from build123d import *

# Parameters (mm, degrees)
CYLINDER074_R             = 11
CYLINDER074_DEPTH         = 10
CYLINDER075_R             = 8
CYLINDER075_DEPTH         = 28
CYLINDER076_R             = 11
CYLINDER076_DEPTH         = 10
CYLINDER083_R             = 1.7
CYLINDER083_DEPTH         = 21
BOX019_W                  = 23
BOX019_H                  = 5.2
BOX019_DEPTH              = 3
PRISM012_DEPTH            = 3
FUSION068_ROLL_ANGLE      = 180
FUSION068_PLACEMENT_ANGLE = 90
EXTRUDE034_DEPTH          = 275
CYLINDER085_R             = 4
CYLINDER085_DEPTH         = 70
PRISM013_DEPTH            = 6
FUSION069_PITCH_ANGLE     = -90
FUSION069_PLACEMENT_ANGLE = -90
CYLINDER073_R             = 11
CYLINDER073_DEPTH         = 10
BOX018_W                  = 34
BOX018_H                  = 24
BOX018_DEPTH              = 6
CYLINDER081_R             = 2.9
CYLINDER081_DEPTH         = 2
CYLINDER082_R             = 2.9
CYLINDER082_DEPTH         = 2
CYLINDER084_R             = 7
CYLINDER084_DEPTH         = 3
EXTRUDE032_DEPTH          = 6
FILLET005_R               = 1.6


with BuildPart() as cilindro074:
    # Cylinder074 → Cylinder074 (new body)
    with BuildSketch(Plane(origin=(83, 3, 55), x_dir=(1, 0, 0), z_dir=(0, 1, 0))):
        Circle(CYLINDER074_R)
    extrude(amount=CYLINDER074_DEPTH)


with BuildPart() as cilindro075:
    # Cylinder075 → Cylinder075 (new body)
    with BuildSketch(Plane(origin=(83, -14, 55), x_dir=(1, 0, 0), z_dir=(0, 1, 0))):
        Circle(CYLINDER075_R)
    extrude(amount=CYLINDER075_DEPTH)


with BuildPart() as cilindro076:
    # Cylinder076 → Cylinder076 (new body)
    with BuildSketch(Plane(origin=(83, -3, 55), x_dir=(1, 0, 0), z_dir=(0, -1, 0))):
        Circle(CYLINDER076_R)
    extrude(amount=CYLINDER076_DEPTH)


with BuildPart() as cilindro083:
    # Cylinder083 → Cylinder083 (new body)
    with BuildSketch(Plane.XY.offset(-6)):
        Circle(CYLINDER083_R)
    extrude(amount=CYLINDER083_DEPTH)


with BuildPart() as cubo018:
    # Box019 → Box019 (new body)
    with BuildSketch(Plane(origin=(0, -2.6, 0), x_dir=(1, 0, 0), z_dir=(0, 0, 1))):
        with Locations((11.5, 2.6)):
            Rectangle(BOX019_W, BOX019_H)
    extrude(amount=BOX019_DEPTH)


with BuildPart() as hueco_tornillo004:
    # Prism012 → Prism012 (new body)
    with BuildSketch(Plane.XY):
        Polygon((3, 0), (1.5, 2.598076), (-1.5, 2.598076), (-3, 0), (-1.5, -2.598076), (1.5, -2.598076), align=None)
    extrude(amount=PRISM012_DEPTH)

    # Fusion068: union Cilindro083, Cubo018
    add(cilindro083.part)
    add(cubo018.part)


with BuildPart() as hueco_tornillo004_1:
    # Fusion068 roll: moved
    add(hueco_tornillo004.part.rotate(Axis((0, 0, 0), (1, 0, 0)), FUSION068_ROLL_ANGLE))


with BuildPart() as hueco_tornillo004_2:
    # Fusion068 placement: moved
    add(hueco_tornillo004_1.part.moved(Location((159, 0, 62))).rotate(Axis((159, 0, 62), (0, 0, 1)), FUSION068_PLACEMENT_ANGLE))


with BuildPart() as extrude034:
    # Sketch026 → Extrude034 (new body)
    with BuildSketch(Plane.YZ):
        with BuildLine():
            ThreePointArc((3.10248, -2.60329), (0, 4.05), (-3.10248, -2.60329))
            Line((-3.10248, -2.60329), (-1.888546, -4.05))
            Line((-1.888546, -4.05), (0, -4.05))
            Line((0, -4.05), (1.888546, -4.05))
            Line((3.10248, -2.60329), (1.888546, -4.05))
        make_face()
    extrude(amount=EXTRUDE034_DEPTH)


with BuildPart() as extrude034_1:
    # Extrude034 placement: moved
    add(extrude034.part.moved(Location((0, 0, 71))))


with BuildPart() as cilindro085:
    # Cylinder085 → Cylinder085 (new body)
    with BuildSketch(Plane.XY):
        Circle(CYLINDER085_R)
    extrude(amount=CYLINDER085_DEPTH)


with BuildPart() as tornillo_m010:
    # Prism013 → Prism013 (new body)
    with BuildSketch(Plane.XY):
        Polygon((7.55, 0), (3.775, 6.538492), (-3.775, 6.538492), (-7.55, 0), (-3.775, -6.538492), (3.775, -6.538492), align=None)
    extrude(amount=PRISM013_DEPTH)

    # Fusion069: union Cilindro085
    add(cilindro085.part)


with BuildPart() as tornillo_m010_1:
    # Fusion069 pitch: moved
    add(tornillo_m010.part.rotate(Axis((0, 0, 0), (0, 1, 0)), FUSION069_PITCH_ANGLE))


with BuildPart() as tornillo_m010_2:
    # Fusion069 placement: moved
    add(tornillo_m010_1.part.moved(Location((203, -7, 55))).rotate(Axis((203, -7, 55), (0, 0, 1)), FUSION069_PLACEMENT_ANGLE))


with BuildPart() as fusion065:
    # Cylinder073 → Cylinder073 (new body)
    with BuildSketch(Plane(origin=(83, -3, 55), x_dir=(1, 0, 0), z_dir=(0, -1, 0))):
        Circle(CYLINDER073_R)
    extrude(amount=CYLINDER073_DEPTH)

    # Fusion065: union Cilindro074, Cilindro075, Cilindro076, hueco_tornillo004, Extrude034, Tornillo_M010
    add(cilindro074.part)
    add(cilindro075.part)
    add(cilindro076.part)
    add(hueco_tornillo004_2.part)
    add(extrude034_1.part)
    add(tornillo_m010_2.part)


with BuildPart() as cubo017:
    # Box018 → Box018 (new body)
    with BuildSketch(Plane(origin=(8, -12, 61), x_dir=(1, 0, 0), z_dir=(0, 0, 1))):
        with Locations((17, 12)):
            Rectangle(BOX018_W, BOX018_H)
    extrude(amount=BOX018_DEPTH)


with BuildPart() as cilindro081:
    # Cylinder081 → Cylinder081 (new body)
    with BuildSketch(Plane(origin=(35, 6, 61), x_dir=(1, 0, 0), z_dir=(0, 0, -1))):
        Circle(CYLINDER081_R)
    extrude(amount=CYLINDER081_DEPTH)


with BuildPart() as cilindro082:
    # Cylinder082 → Cylinder082 (new body)
    with BuildSketch(Plane(origin=(15, -6, 61), x_dir=(1, 0, 0), z_dir=(0, 0, -1))):
        Circle(CYLINDER082_R)
    extrude(amount=CYLINDER082_DEPTH)


with BuildPart() as cilindro084:
    # Cylinder084 → Cylinder084 (new body)
    with BuildSketch(Plane(origin=(203, 6, 55), x_dir=(1, 0, 0), z_dir=(0, 1, 0))):
        Circle(CYLINDER084_R)
    extrude(amount=CYLINDER084_DEPTH)


with BuildPart() as fillet005:
    # Sketch024 → Extrude032 (new body, symmetric)
    with BuildSketch(Plane.XZ):
        with BuildLine():
            Line((8, 77), (218, 77))
            Line((218, 77), (218, 61.5))
            Line((218, 61.5), (212.987446, 50.640129))
            ThreePointArc((193.012554, 50.640129), (203, 44.25), (212.987446, 50.640129))
            Line((193.012554, 50.640129), (189.340668, 58.595396))
            ThreePointArc((189.340668, 58.595396), (187.495639, 60.711709), (184.80092, 61.5))
            Line((165, 61.5), (184.80092, 61.5))
            Line((165, 56.5), (165, 61.5))
            Line((153, 56.5), (165, 56.5))
            Line((153, 61.5), (153, 56.5))
            Line((109.772187, 61.5), (153, 61.5))
            ThreePointArc((109.772187, 61.5), (103.17533, 59.015416), (99.856562, 52.796296))
            ThreePointArc((66.143438, 52.796296), (83, 38), (99.856562, 52.796296))
            ThreePointArc((66.143438, 52.796296), (62.82467, 59.015416), (56.227813, 61.5))
            Line((8, 61.5), (56.227813, 61.5))
            Line((8, 77), (8, 61.5))
        make_face()
    extrude(amount=EXTRUDE032_DEPTH, both=True)

    # Fusion066: union Cubo017, Cilindro081, Cilindro082, Cilindro084
    add(cubo017.part)
    add(cilindro081.part)
    add(cilindro082.part)
    add(cilindro084.part)

    # Cut024: cut Fusion065
    add(fusion065.part, mode=Mode.SUBTRACT)

    # Fillet005
    fillet005_edges = [fillet005.edges().sort_by_distance(p)[0] for p in [
        (218, 6, 69.25),
        (215.493723, 6, 56.070064),
        (49.113906, 6, 61.5),
        (203, 6, 44.25),
        (62.82467, 6, 59.015416),
        (191.176611, 6, 54.617762),
        (83, 6, 38),
        (187.495639, 6, 60.711709),
        (103.17533, 6, 59.015416),
        (174.90046, 6, 61.5),
        (131.386094, 6, 61.5),
        (165, 6, 59),
        (153, 6, 59),
        (159, 6, 56.5),
        (218, -6, 69.25),
        (42, 12, 64),
        (42, -12, 64),
        (215.493723, -6, 56.070064),
        (203, -6, 44.25),
        (62.82467, -6, 59.015416),
        (191.176611, -6, 54.617762),
        (83, -6, 38),
        (187.495639, -6, 60.711709),
        (103.17533, -6, 59.015416),
        (174.90046, -6, 61.5),
        (131.386094, -6, 61.5),
        (165, 0, 56.5),
        (165, -6, 59),
        (153, 0, 56.5),
        (153, -6, 59),
        (159, -6, 56.5),
    ]]
    fillet(fillet005_edges, radius=FILLET005_R)


solid = fillet005.part
Source: CAD feature listing. Evaluate the final solid. Frame: model axes, mm. A direction names the side the tool comes from. Round coordinates to 2 decimals unless told otherwise and drop trailing zeros. Order: outer loops, then holes, each group sorted by start corner. A loop starts at its lowest first (then second) coordinate and runs counter-clockwise, first axis right, second up. Notation, with made-up numbers: (56, -2) - (95, -2) arc R33 cw to (95, 36) - close; hole circle Ø5 at (43.5, 30). An arc over 180 degrees is marked (long way). Use a Markdown table: item, result. Add a question column.
1. Section query A-A (x = 83). Return the cut outline in (y, z), then the cut area to 3 significant figures.
2. Set-up query: faces 1 (the cylindrical face through (12.1, -6.1, 60)), 2 (the cylindrical face through (72, 4, 55)), 3 (the flat face through (209.538, -4, 55)). Return all of +Z, -Z, +X, -X, +Y, -Y with unobstructed straight access to the full face (end or side cutting, diameter ignored); none if empty.
3. Line query: probe 1 along Y at (x, z) = (100, 71); probe 2 along X at (y, z) = (0, 64.9); probe 3 along X at (y, z) = (5.2, 55). Output: solid intervals per line, ascending.
4. First-contact query: pin 1 (1.5 mm diameter, centred on x = 121, y = 6, fed in from -Z); pin 2 (2.5 mm diameter, centred on y = -3, z = 57, fed in from +X); pin 3 (1.5 mm diameter, centred on y = -6.5, z = 57.5, fed in from +X). Flat tips, straight axial feed; report the tip coordinate or a pass-through.
5. Section query D-D (x = 145). Return the cut outline in (y, z), then the cut area to 3 significant figures.
6. Section query B-B (z = 71). Return the cut outline in (x, y), then the cut area to 3 significant figures.
7. Mould query, pull axis Z, two halves, no side actions, for faces 4 (the flat face through (25, 9, 67)), 5 (the cylindrical face through (157.34, -0.37, 57.77)), 6 (the flat face through (159, 2, 62)). Classes: +Z half, -Z half, draft (parallel to the pull), parting line (faces both ways), or undercut.
8. Section query C-C (x = 35). Return the cut outline in (y, z).
Derived:
| question | item | result |
|---|---|---|
| 1 | outline | (-6, 39.6) arc R1.6 ccw to (-4.4, 38) - (4.4, 38) arc R1.6 ccw to (6, 39.6) - (6, 44) - (3, 44) - (3, 47) - (-3, 47) - (-3, 44) - (-6, 44) - close; (-6, 66) - (-3, 66) - (-3, 63) - (3, 63) - (3, 66) - (6, 66) - (6, 77) - (-6, 77) - close; hole (-3.1, 68.4) - (-1.89, 66.95) - (1.89, 66.95) - (3.1, 68.4) arc R4.05 ccw (long way) to start |
| 1 | area | 186 mm2 |
| 2 | face 1 | -Z |
| 2 | face 2 | +Y |
| 2 | face 3 | -Y |
| 3 | probe 1 | -6 to -4.05, 4.05 to 6 |
| 3 | probe 2 | 8 to 157.3, 160.7 to 218 |
| 3 | probe 3 | 65.82 to 72, 94 to 100.18, 191.24 to 199, 207 to 214.76 |
| 4 | pin 1 | z = 61.74 |
| 4 | pin 2 | x = 216.5 |
| 4 | pin 3 | x = 215.38 |
| 5 | outline | (-6, 63.1) arc R1.6 ccw to (-4.4, 61.5) - (4.4, 61.5) arc R1.6 ccw to (6, 63.1) - (6, 77) - (-6, 77) - close; hole (-3.1, 68.4) - (-1.89, 66.95) - (1.89, 66.95) - (3.1, 68.4) arc R4.05 ccw (long way) to start |
| 5 | area | 132 mm2 |
| 6 | outline | (8, -6) - (216.4, -6) arc R1.6 ccw to (218, -4.4) - (218, -4.05) - (8, -4.05) - close; (8, 4.05) - (218, 4.05) - (218, 4.4) arc R1.6 ccw to (216.4, 6) - (8, 6) - close |
| 6 | area | 818 mm2 |
| 7 | face 4 | +Z half |
| 7 | face 5 | draft |
| 7 | face 6 | undercut |
| 8 | outline | (-12, 61) - (3.1, 61) - (3.1, 59) - (8.9, 59) - (8.9, 61) - (12, 61) - (12, 67) - (6, 67) - (6, 77) - (-6, 77) - (-6, 67) - (-12, 67) - close; hole (-3.1, 68.4) - (-1.89, 66.95) - (1.89, 66.95) - (3.1, 68.4) arc R4.05 ccw (long way) to start |
